The drawing under review shows one solid part. Ordinate dimensions are in mm from its lowest x, y, z. A direction names the side the tool comes from. Coordinates: 2 decimals unless noted, no trailing zeros. Write each loop counter-clockwise with the first axis right and the second up, starting at its lowest first coordinate (ties: lowest second). Pieces come first, ordered by that corner, then holes. Notation, with made-up numbers: (-7.75, 9.25) - (12.25, 9.25) arc R27 ccw to (12.25, 40.25) - close; hole circle Ø5 at (68, 60). An arc over 180 degrees is marked (long way). Use a Markdown table: item, result.
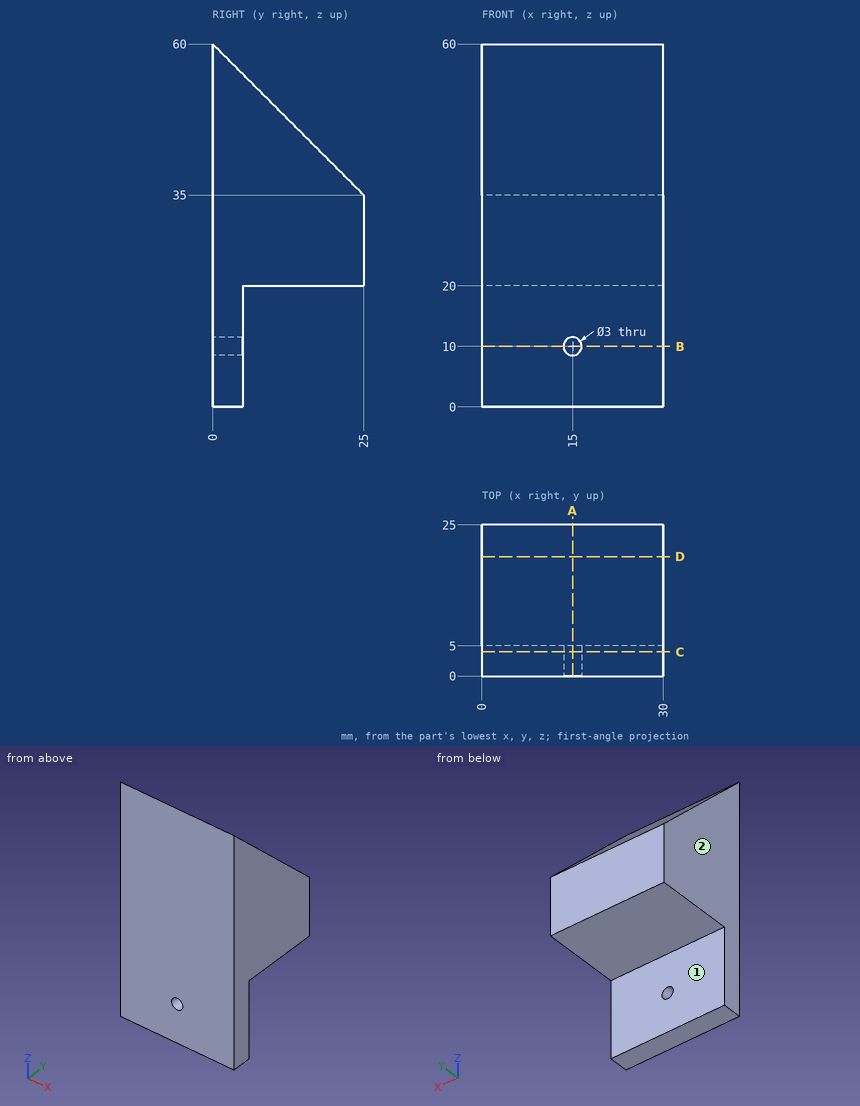
(1) Take a section at B-B on z = 10. Write out the cut boundary in (x, y).
Determined:
| item | result |
|---|---|
| outline | (0, 0) - (13.5, 0) - (13.5, 5) - (0, 5) - close; (16.5, 0) - (30, 0) - (30, 5) - (16.5, 5) - close |
(2) Take a section at C-C on y = 4. Write out the cut boundary in (x, z), and give its area (3 significant figures).
Determined:
| item | result |
|---|---|
| outline | (0, 0) - (30, 0) - (30, 56) - (0, 56) - close; hole circle Ø3 at (15, 10) |
| area | 1,670 mm2 |
(3) Take a section at D-D on y = 19.75. Write out the cut boundary in (x, z), and give its area (4 significant figures).
Determined:
| item | result |
|---|---|
| outline | (0, 20) - (30, 20) - (30, 40.25) - (0, 40.25) - close |
| area | 607.5 mm2 |
(4) Machinability: for the marked faces 1 and 2, which of the approach directions +Z, -Z, +X, -X, +Y, -Y give a long, thin tool a straight path to every point of the face, cutting with its end or side? Answer none if there is none.
Determined:
| item | result |
|---|---|
| face 1 | -Z, +X, -X, +Y |
| face 2 | +Z, -Z, -X, +Y, -Y |
(5) For L1, parallel to X at y = 3.15, z = 10; L2, parallel to Y at x = 18.75, z = 12; L3, parallel to Y at x = 6, z = 40, list the stretches that pass through material, from the lowest coordinate up. Write a range as from..to.
Determined:
| item | result |
|---|---|
| L1 | 0..13.5, 16.5..30 |
| L2 | 0..5 |
| L3 | 0..20 |
(6) Take a section at A-A on x = 15. Write out the cut boundary in (y, z), and give its area (4 significant figures).
Determined:
| item | result |
|---|---|
| outline | (0, 0) - (5, 0) - (5, 8.5) - (0, 8.5) - close; (0, 11.5) - (5, 11.5) - (5, 20) - (25, 20) - (25, 35) - (0, 60) - close |
| area | 772.5 mm2 |
(7) For pin 1 (2 mm diameter, centred on x = 23.5, y = 19.5, fed in from -Z); pin 2 (12 mm diameter, centred on x = 5.5, y = 10.5, fed in from +Z); pin 3 (1 mm diameter, centred on x = 25, y = 11.5, fed in from +Z), all flat-tipped, find the tip position at first contact; note any pin that passes through.
Determined:
| item | result |
|---|---|
| pin 1 | z = 20 |
| pin 2 | z = 55.5 |
| pin 3 | z = 49 |
